```python
from build123d import *

# Parameters (mm, degrees)
SKETCH1_W                  = 76.2
SKETCH1_H                  = 9.525
BOSS_EXTRUDE1_DEPTH        = 39.624
FILLET1_R                  = 12.7
SKETCH2_R                  = 2.54
CUT_EXTRUDE1_DEPTH         = 87.018502558
SKETCH3_W                  = 32.004
SKETCH3_H                  = 9.525
BOSS_EXTRUDE2_DEPTH        = 53.975
FILLET2_R                  = 16.002
FILLET3_R                  = 16.002
SKETCH4_R                  = 16.002
BOSS_EXTRUDE3_DEPTH        = 14.097
BOSS_EXTRUDE4_DEPTH        = 4.826
SKETCH6_R                  = 6.35
CUT_EXTRUDE2_DEPTH         = 89.301196715
F_3_8_0_5_DIAMETER_HOLE1_D = 12.7


with BuildPart() as part:
    # Sketch1 → Boss-Extrude1 (new body)
    with BuildSketch(Plane.XY):
        Rectangle(SKETCH1_W, SKETCH1_H)
    extrude(amount=BOSS_EXTRUDE1_DEPTH)

    # Fillet1
    fillet1_edges = [part.edges().sort_by_distance(p)[0] for p in [
        (-38.1, 0, 39.624),
        (38.1, 0, 39.624),
    ]]
    fillet(fillet1_edges, radius=FILLET1_R)

    # Sketch2 → Cut-Extrude1 (cut, through all)
    with BuildSketch(Plane(origin=(38.1, 0, 0), x_dir=(0, 0, -1), z_dir=(1, 0, 0))):
        with Locations((0, 4.7625)):
            Circle(SKETCH2_R)
    extrude(amount=-CUT_EXTRUDE1_DEPTH, mode=Mode.SUBTRACT)

    # Sketch3 → Boss-Extrude2 (add)
    with BuildSketch(Plane(origin=(0, 4.7625, 0), x_dir=(1, 0, 0), z_dir=(0, 1, 0))):
        with Locations((0, -7.3025)):
            Rectangle(SKETCH3_W, SKETCH3_H)
    extrude(amount=BOSS_EXTRUDE2_DEPTH)

    # Fillet2
    fillet2_edges = [part.edges().sort_by_distance(p)[0] for p in [
        (-16.002, 4.7625, 7.3025),
    ]]
    fillet(fillet2_edges, radius=FILLET2_R)

    # Fillet3
    # the kernel refuses this fillet: 16.002 mm, written as the material it adds along each edge
    with BuildSketch(Plane(origin=(16.002, 4.7625, 2.54), x_dir=(0, 1, 0), z_dir=(0, 0, 1))) as fillet3_piece_1:
        with BuildLine():
            CenterArc((FILLET3_R, -FILLET3_R), FILLET3_R, 90, 90)
            Line((0, -FILLET3_R), (0, 0))
            Line((0, 0), (FILLET3_R, 0))
        make_face()
    extrude(amount=9.525)

    # Sketch4 → Boss-Extrude3 (add)
    with BuildSketch(Plane.XY.offset(12.065)):
        with Locations((0, 58.7375)):
            Circle(SKETCH4_R)
    extrude(amount=-BOSS_EXTRUDE3_DEPTH)

    # Sketch5 → Boss-Extrude4 (add, symmetric)
    with BuildSketch(Plane(origin=(0, 0, 0), x_dir=(0, 0, -1), z_dir=(1, 0, 0))):
        Polygon((-39.624, 4.7625), (-12.065, 4.7625), (-12.065, 46.0375), align=None)
    extrude(amount=BOSS_EXTRUDE4_DEPTH, both=True)

    # Sketch6 → Cut-Extrude2 (cut, through all)
    with BuildSketch(Plane.XY.offset(12.065)):
        with Locations((0, 58.7375)):
            Circle(SKETCH6_R)
    extrude(amount=-CUT_EXTRUDE2_DEPTH, mode=Mode.SUBTRACT)

    # 3/8 (0.5) Diameter Hole1 (through all)
    with Locations(Plane(origin=(0, 4.7625, 0), x_dir=(1, 0, 0), z_dir=(0, 1, 0))):
        with Locations((-25.4, -26.924), (25.4, -26.924)):
            Hole(F_3_8_0_5_DIAMETER_HOLE1_D / 2)


solid = part.part
```
Geometry check sheet. Reference: the model listing, model coordinates, mm. A direction names the side the tool comes from. Give positions to 0.01 mm unless a question says otherwise; leave off trailing zeros. Write each loop counter-clockwise with the first axis right and the second up, starting at its lowest first coordinate (ties: lowest second). Pieces come first, ordered by that corner, then holes. Notation, with made-up numbers: (1, 39.25) -> (40, 39.25) arc R30 ccw to (40, 73.25) -> close; hole circle Ø5 at (57, 20). An arc over 180 degrees is marked (long way). One line per question, with ' | ' between items.
Item 1: Sectioned sample at D-D, the plane z = 16. Record the boundary of the cut face in (x, y), plus the area to 3 significant figures.
Determined:
outline: (-38.1, -4.76) -> (38.1, -4.76) -> (38.1, 4.76) -> (4.83, 4.76) -> (4.83, 40.14) -> (-4.83, 40.14) -> (-4.83, 4.76) -> (-38.1, 4.76) -> close | area: 1,070 mm^2
Item 2: Sectioned sample at B-B, the plane x = 0. Record the boundary of the cut face in (y, z) (1 decimal).
Determined:
outline: (-4.8, 0) -> (2.2, 0) arc R2.5 cw to (4.8, 2.5) -> (42.7, 2.5) -> (42.7, -2) -> (52.4, -2) -> (52.4, 12.1) -> (46, 12.1) -> (4.8, 39.6) -> (-4.8, 39.6) -> close; (65.1, -2) -> (74.7, -2) -> (74.7, 12.1) -> (65.1, 12.1) -> close
Item 3: Sectioned sample at C-C, the plane y = 0.5. Record the boundary of the cut face in (x, z).
Determined:
outline: (-38.1, 0) -> (38.1, 0) -> (38.1, 26.92) arc R12.7 ccw to (25.4, 39.62) -> (-25.4, 39.62) arc R12.7 ccw to (-38.1, 26.92) -> close; hole circle Ø12.7 at (-25.4, 26.92); hole circle Ø12.7 at (25.4, 26.92)
Item 4: Scan lines: line 1 along Z through (x, y) = (-25.4, 0); line 2 along Y through (x, z) = (0, 8); line 3 along Y through (x, z) = (-20, 37). Record each from-to range of solid material in increasing order.
Determined:
line 1: 0 to 20.57, 33.27 to 39.62 | line 2: -4.76 to 52.39, 65.09 to 74.74 | line 3: -4.76 to 4.76
Item 5: Sectioned sample at A-A, the plane z = 10. Record the boundary of the cut face in (x, y), plus the area to 3 significant figures.
Determined:
outline: (-38.1, -4.76) -> (38.1, -4.76) -> (38.1, 4.76) -> (32, 4.76) arc R16 cw to (16, 20.76) -> (16, 58.74) arc R16 ccw to (-16, 58.74) -> (-16, 20.76) arc R16 cw to (-32, 4.76) -> (-38.1, 4.76) -> close; hole circle Ø12.7 at (0, 58.74) | area: 2,840 mm^2
Item 6: Depth check by flat-ended pin: pin 1 (22 mm diameter, centred on y = 30.5, z = 21, fed in from -X); pin 2 (4 mm diameter, centred on y = 21.5, z = 23, fed in from -X); pin 3 (7.5 mm diameter, centred on y = 31, z = 8.5, fed in from +X); pin 4 (8 mm diameter, centred on x = -23.5, y = 38.5, fed in from +Z). Enter the tip coordinate at first touch or a pass-through.
Determined:
pin 1: x = -16 | pin 2: x = -4.83 | pin 3: x = 16 | pin 4: through
Item 7: Draft check along Z on faces 4 (the cylindrical face through (-20.36, -0.07, 30.79)), 5 (the cylindrical face through (-2.1, 74.6, 3.5)), 6 (the flat face through (0.07, 25.69, 25.65)). Enter one of: released by +Z, released by -Z, zero draft, split by the parting line, or undercut.
Determined:
face 4: undercut | face 5: zero draft | face 6: released by +Z
Item 8: Access from +Z, -Z, +X, -X, +Y, -Y to the whole of each face (thin tool, end or side, straight path). Record for faces 1 (the flat face through (21, 4.762, 21)), 2 (the flat face through (7, 40, 12.065)), 3 (the cylindrical face through (0.53, 2.99, 1.82)).
Determined:
face 1: +Z, +X, +Y | face 2: +Z, +Y | face 3: -Z, +X, -X
